Autodesk Inventor part; units mm, degrees
ref_plane "Work Plane7" through (0, 5.08, 0) normal (0, 1, 0) x (1, 0, 0)
ref_plane "YZ Plane" through (0, 0, 0) normal (1, 0, 0) x (0, 1, 0)
ref_plane "XZ Plane" through (0, 0, 0) normal (0, 1, 0) x (-1, 0, 0)
ref_plane "Work Plane7" through (0, 5.08, 0) normal (0, 1, 0) x (1, 0, 0)
sketch "Sketch3" plane through (0, 5.08, 0) normal (0, 1, 0) x (1, 0, 0)
  circle A0 centre (0, 0) radius 6.5659
  circle A1 centre (0, 0) radius 3.3655
  line L0 (-6.5659, 0) -> (-6.5659, -6.5683)
  line L1 (-6.5659, -6.5683) -> (6.5659, -6.5683)
  line L2 (6.5659, -6.5683) -> (6.5659, 0)
  line L3 (0, -6.5683) -> (0, -9.1083)
  line L4 (0, 0) -> (0, -9.1083) construction
  line L5 (6.5659, 0) -> (6.5659, -9.1083)
  line L6 (-6.5659, -9.1083) -> (-6.5659, 0)
  arc A2 (6.5659, 0) -> (-6.5659, 0) centre (0, 0) ccw
  arc A3 (-6.5659, -9.1083) -> (6.5659, -9.1083) centre (0, -9.1083) ccw
  line L7 (0, -6.5683) -> (0, -7.8383)
  arc A4 (-6.5659, -4.2811) -> (6.5659, -4.2811) centre (0, 0) ccw
  point P0 (0, -4.5541)
  dimension "d19" = 2.54
  dimension "d20" = 1.27
extrude "Extrusion5" add sketch "Sketch3" along normal blind 2.54 contours A0 | L2 A4 L1 L0 A0 | L2 L1 A4 | A4 L1 L0 | L5 A3 L6 L1 A4 | A4 L3 L1 | L1 L3 A4 | A1
extrude "Extrusion6" add sketch "Sketch3" along normal blind 7.62
sketch "Sketch4" plane through (0, 12.7, 0) normal (0, 1, 0) x (1, 0, 0)
  line L0 (-6.5659, 0) -> (-6.5659, -9.1083)
  arc A0 (-6.5659, -9.1083) -> (6.5659, -9.1083) centre (0, -9.1083) ccw
  line L1 (6.5659, -9.1083) -> (6.5659, 0)
  arc A1 (6.5659, 0) -> (-6.5659, 0) centre (0, 0) ccw
  circle A2 centre (0, 0) radius 3.3655
  line L2 (0, -3.3655) -> (0, -7.1755)
  line L3 (0, -7.1755) -> (6.5659, -7.1755)
  line L4 (0, -7.1755) -> (-6.5659, -7.1755)
  arc A3 (-6.5659, -2.8943) -> (6.5659, -2.8943) centre (0, 0) ccw
  line L5 (0, -9.1083) -> (0, -7.1755)
  line L6 (0, -7.1755) -> (0, -7.8105)
  arc A4 (-6.5659, -4.23) -> (6.5659, -4.23) centre (0, 0) ccw
  dimension "d25" = 3.81
  dimension "d27" = 0.635
extrude "Extrusion7" add sketch "Sketch4" along normal blind 52.07 contours A4 L4 L0 | L4 A4 L3 L1 A0 L0 | A4 L1 L3
fillet "Fillet1" radius 1.27 2 edges at (6.5659, 38.735, 4.23) (-6.5659, 38.735, 4.23)
sketch "Sketch5" plane through (0, 64.77, 0) normal (0, 1, 0) x (1, 0, 0)
  arc A0 (-4.5552, -6.3446) -> (-6.5659, -7.3762) centre (-5.2959, -7.3762) ccw
  line L0 (-6.5659, -7.3762) -> (-6.5659, -9.1083)
  arc A1 (-6.5659, -9.1083) -> (6.5659, -9.1083) centre (0, -9.1083) ccw
  line L1 (6.5659, -9.1083) -> (6.5659, -7.3762)
  arc A2 (6.5659, -7.3762) -> (4.5552, -6.3446) centre (5.2959, -7.3762) ccw
  arc A3 (-4.5552, -6.3446) -> (4.5552, -6.3446) centre (0, 0) ccw
  arc A4 (-4.5552, -6.3446) -> (4.5552, -6.3446) centre (0, 0) ccw
  arc A5 (6.5659, -7.3762) -> (4.5552, -6.3446) centre (5.2959, -7.3762) ccw
  line L2 (6.5659, -7.3762) -> (6.5659, 0)
  arc A6 (6.5659, 0) -> (-6.5659, 0) centre (0, 0) ccw
  line L3 (-6.5659, 0) -> (-6.5659, -7.3762)
  arc A7 (-4.5552, -6.3446) -> (-6.5659, -7.3762) centre (-5.2959, -7.3762) ccw
  circle A8 centre (0, 0) radius 3.3655
  circle A9 centre (0, 0) radius 3.4925
  line L4 (0, -9.1083) -> (0, -11.0133)
  line L5 (5.2959, -7.3762) -> (0, -11.0133)
  line L6 (-5.2959, -7.3762) -> (0, -11.0133)
  line L7 (0, -11.0133) -> (0, -11.6483)
  circle A10 centre (0, -11.6483) radius 1.905
  point P0 (6.5659, -7.3762)
  dimension "d31" = 6.985
  dimension "d32" = 1.905
  dimension "d34" = 0.635
  dimension "d35" = 3.81
extrude "Extrusion8" add sketch "Sketch5" along normal blind 7.62 contours A3 A2 L1 A1 L0 A0 | A0 L3 A6 L2 A2 A3
extrude "Extrusion9" cut sketch "Sketch5" against normal blind 7.62 contours A10 L5 L4 | L4 L6 A10 | L5 A10 L6
sketch "Sketch6" plane through (0, 72.39, 0) normal (0, 1, 0) x (1, 0, 0)
  arc A0 (6.5659, 0) -> (-6.5659, 0) centre (0, 0) ccw
  line L0 (-6.5659, 0) -> (-6.5659, -9.1083)
  arc A1 (-6.5659, -9.1083) -> (6.5659, -9.1083) centre (0, -9.1083) ccw
  line L1 (6.5659, -9.1083) -> (6.5659, 0)
  circle A2 centre (0, -11.6483) radius 1.905
  circle A3 centre (0, 0) radius 3.4925
extrude "Extrusion10" add sketch "Sketch6" against normal blind 12.7
extrude "Extrusion11" cut sketch "Sketch6" against normal blind 5.08
sketch "Sketch7" plane through (0, 57.15, 11.6483) normal (0, 1, 0) x (1, 0, 0)
  circle A0 centre (0, 0) radius 1.905
  point P0 (0, 11.6483)
extrude "Extrusion12" add sketch "Sketch7" along normal blind 2.54
properties part number "Odometer_Test_Bracket"
Can you work these out from the model? Positions are in its coordinate system, mm. A direction names the side the tool comes from. Round coordinates to 2 decimals unless told otherwise and drop trailing zeros. Loops run counter-clockwise (first coordinate to the right, second up) from the corner with the lowest first, then second, coordinate; pieces in that order, holes last. Notation, with made-up numbers: (30, 51) - (54, 51) arc R16 cw to (54, 71) - close; hole circle Ø3 at (15, 57). An arc over 180 degrees is marked (long way). Answer in a Markdown table with one row per item. Add a question column.
Q1. Which directions (+Z, -Z, +X, -X, +Y, -Y) give clear straight access to the entire face, cutting with the end or side of a thin tool? Please do faces 1 (the cylindrical face through (-0.413, 63.447, 9.789)), 2 (the cylindrical face through (5.893, 36.524, 6.255)), 3 (the cylindrical face through (-0.144, 8.837, -6.564)).
Q2. For pin 1 Ø1 at (x, y) = (-1, 19.5) entering from -Z; pin 2 Ø8 at (y, z) = (48, 12.5) entering from +X; pin 3 Ø1.1 at (x, z) = (-0.5, 11.5) entering from +Y; pin 4 Ø4 at (y, z) = (43, 4.5) entering from -X, each with a flat end and sliding along its axis, tell me the tip position at first contact or that it passes through.
Q3. I want a section at C-C on y = 37. List the corners of the cut face in (x, z) for me.
Q4. I want a section at B-B on z = -2.75. List the corners of the cut face in (x, y) for me, and give its area (3 significant figures).
Q5. I want a section at A-A on x = 0. List the corners of the cut face in (y, z) for me.
Q6. We'd pull the mould along Y, two halves only. Please class faces 4 (the flat face through (0, 12.7, 4)), 5 (the flat face through (0, 7.62, 0)), 6 (the cylindrical face through (0.144, 35.759, 15.673)): pulls with the +Y half, pulls with the -Y half, needs draft (parallel to the pull), parting line crosses it, or undercut.
Q7. I need wall thicknesses on L1, parallel to Z at x = 0, y = 61.75; L2, parallel to X at y = 12, z = -0.25; L3, parallel to Z at x = 0, y = 11.75. Which ranges of each line are inside material? Lowest first, please.
Q8. I want a section at D-D on x = -2.5. List the corners of the cut face in (y, z) for me, and give its area (3 significant figures).
A:
| question | item | result |
|---|---|---|
| 1 | face 1 | +Y |
| 1 | face 2 | -Z |
| 1 | face 3 | -Z, +Y, -Y |
| 2 | pin 1 | z = 7.67 |
| 2 | pin 2 | x = 6.57 |
| 2 | pin 3 | y = 59.69 |
| 2 | pin 4 | x = -6.22 |
| 3 | outline | (-6.57, 7.38) arc R1.27 ccw to (-4.56, 6.34) arc R7.81 cw to (4.56, 6.34) arc R1.27 ccw to (6.57, 7.38) - (6.57, 9.11) arc R6.57 ccw to (-6.57, 9.11) - close |
| 4 | outline | (-5.96, 5.08) - (5.96, 5.08) - (5.96, 12.7) - (1.94, 12.7) - (1.94, 7.62) - (-1.94, 7.62) - (-1.94, 12.7) - (-5.96, 12.7) - close; (-5.96, 59.69) - (-2.15, 59.69) - (-2.15, 67.31) - (-5.96, 67.31) - close; (2.15, 59.69) - (5.96, 59.69) - (5.96, 67.31) - (2.15, 67.31) - close |
| 4 | area | 129 mm^2 |
| 5 | outline | (5.08, -6.57) - (12.7, -6.57) - (12.7, -3.37) - (7.62, -3.37) - (7.62, 3.37) - (12.7, 3.37) - (12.7, 7.81) - (59.69, 7.81) - (59.69, 3.49) - (67.31, 3.49) - (67.31, 9.74) - (59.69, 9.74) - (59.69, 13.55) - (67.31, 13.55) - (67.31, 15.67) - (5.08, 15.67) - close; (59.69, -6.57) - (67.31, -6.57) - (67.31, -3.49) - (59.69, -3.49) - close |
| 6 | face 4 | undercut |
| 6 | face 5 | pulls with the +Y half |
| 6 | face 6 | needs draft |
| 7 | L1 | -6.57 to -3.49, 3.49 to 9.74, 13.55 to 15.67 |
| 7 | L2 | -6.56 to -3.36, 3.36 to 6.56 |
| 7 | L3 | -6.57 to -3.37, 3.37 to 15.67 |
| 8 | outline | (5.08, -6.07) - (12.7, -6.07) - (12.7, -2.25) - (7.62, -2.25) - (7.62, 2.25) - (12.7, 2.25) - (12.7, 7.4) - (59.69, 7.4) - (59.69, 2.44) - (67.31, 2.44) - (67.31, 15.18) - (5.08, 15.18) - close; (59.69, -6.07) - (67.31, -6.07) - (67.31, -2.44) - (59.69, -2.44) - close |
| 8 | area | 629 mm^2 |
